The listing builds one solid part. Answer for the finished solid, in the listing's coordinates (mm). A direction names the side the tool comes from. Coordinates: 2 decimals unless noted, no trailing zeros. Order: outer loops, then holes, each group sorted by start corner. A loop starts at its lowest first (then second) coordinate and runs counter-clockwise, first axis right, second up. Notation, with made-up numbers: (22.5, 86.5) -> (49.5, 86.5) arc R18 ccw to (49.5, 106.5) -> close; hole circle Ø8 at (77.5, 80.5). An arc over 180 degrees is marked (long way). Return JSON: item names as keys, results as strings.
from build123d import *

# Parameters (mm, degrees)
F2_R     = 12.7
F3_DEPTH = 25.4
F7_R     = 12.7
F8_DEPTH = 25.4


# Not quite as in the source:
# - the program builds the solid bodies; features that only make, move or delete a surface that nothing else refers to are left out


with BuildPart() as f1:
    # F0 (on Front) → F1 (revolve)
    with BuildSketch(Plane.XZ):
        with BuildLine():
            ThreePointArc((0, -12.7), (8.9802561211, -8.9802561211), (12.7, 0))
            ThreePointArc((12.7, 0), (8.9802561211, 8.9802561211), (0, 12.7))
            Line((0, 12.7), (0, -12.7))
        make_face()
    revolve(axis=Axis((0, 0, -1.3322243467), (0, 0, -1)))

    # F2 (on Right) → F3 (join)
    with BuildSketch(Plane.YZ):
        Circle(F2_R)
    extrude(amount=F3_DEPTH)

    # F7 (on Top) → F8 (join)
    with BuildSketch(Plane.XY):
        Circle(F7_R)
    extrude(amount=F8_DEPTH)


solid = f1.part
1. The part is cut by section A-A on y = 0. Give the vertices of the cut face in (x, z), and give its area (3 significant figures).
Answer block:
{"outline": "(-12.7, 0) arc R12.7 ccw to (0, -12.7) -> (25.4, -12.7) -> (25.4, 12.7) -> (12.7, 12.7) -> (12.7, 25.4) -> (-12.7, 25.4) -> close", "area": "1,260 mm2"}
2. The part is cut by section B-B on x = 7.5. Give the vertices of the cut face in (y, z).
Answer block:
{"outline": "(-10.25, 7.5) arc R12.7 ccw (long way) to (10.25, 7.5) -> (10.25, 25.4) -> (-10.25, 25.4) -> close"}
3. Consider line 1 (Y direction, x = 1.5, z = 0.5); line 2 (X direction, y = -9.5, z = 17.5). Determine where each line is inside the solid, lowest interval first. Write a range as from..to.
Answer block:
{"line 1": "y = -12.69..12.69", "line 2": "x = -8.43..8.43"}
4. Each of these flat-tipped pins is pushed along its axis until it touches: pin 1 Ø4 at (x, z) = (20, 11) entering from -Y; pin 2 Ø5 at (x, z) = (6, 7) entering from -Y; pin 3 Ø4 at (x, z) = (12.5, 21) entering from -Y. Where does it stop, or does it pass through?
Answer block:
{"pin 1": "stops at y = -8.96", "pin 2": "stops at y = -12.21", "pin 3": "stops at y = -7.14"}
5. The part is cut by section C-C on y = 8. Give the vertices of the cut face in (x, z), and give its area (3 significant figures).
Answer block:
{"outline": "(-9.86, 0) arc R9.86 ccw to (0, -9.86) -> (25.4, -9.86) -> (25.4, 9.86) -> (9.86, 9.86) -> (9.86, 25.4) -> (-9.86, 25.4) -> close", "area": "981 mm2"}
6. For faces 1 (the face through (12.52, -2.75, -12.4)), 2 (the face through (0, 0, 25.4)), 3 (the face through (-12.688, 0.558, 12.522)), determine the directions among +Z, -Z, +X, -X, +Y, -Y from which every point of the face is accessible in a straight line to the end or side of a thin tool.
Answer block:
{"face 1": "+X", "face 2": "+Z, +X, -X, +Y, -Y", "face 3": "+Z"}
7. The part is cut by section D-D on z = -7.5. Give the vertices of the cut face in (x, y).
Answer block:
{"outline": "(0, -10.25) -> (25.4, -10.25) -> (25.4, 10.25) -> (0, 10.25) arc R10.25 ccw to start"}
